Autodesk Inventor part; units mm, degrees
ref_plane "YZ Plane" through (0, 0, 0) normal (1, 0, 0) x (0, 1, 0)
ref_plane "XZ Plane" through (0, 0, 0) normal (0, 1, 0) x (-1, 0, 0)
ref_plane "XY Plane" through (0, 0, 0) normal (0, 0, 1) x (1, 0, 0)
sketch "Sketch1" plane through (0, 0, 0) normal (1, 0, 0) x (0, 1, 0)
  circle A0 centre (0, 0) radius 13.5
  dimension "d0" = 27
extrude "Extrusion1" add sketch "Sketch1" along normal blind 106
sketch "Sketch2" plane through (106, 0, 0) normal (1, 0, 0) x (0, 0, -1)
  circle A0 centre (0, 0) radius 1.5
  dimension "d3" = 3
extrude "Extrusion2" add sketch "Sketch2" along normal blind 12 and the other way blind 112.25
properties part number "ROLLER"
Source: CAD feature listing. Evaluate the final solid. Frame: model axes, mm. A direction names the side the tool comes from. Coordinates: 2 decimals unless noted, no trailing zeros. Loops run counter-clockwise (first coordinate to the right, second up) from the corner with the lowest first, then second, coordinate; pieces in that order, holes last. Notation, with made-up numbers: M 34,2 L 69,2 A20 cw 69,39 Z; hole C -30.75,-39 d8. An arc over 180 degrees is marked long. Put each result on its own line as item: value. Start each with the question number.
1) Cut plane A-A on y = 0. Return the cut outline in (x, z), then the cut area to 3 significant figures.
2) Cut plane C-C on x = 22. Return the cut outline in (y, z).
3) Cut plane D-D on y = 8.75. Return the cut outline in (x, z), then the cut area to 3 significant figures.
4) Pull-direction query (Z, two-part tool) for faces 1 (the face through (0, 3, 0)), 2 (the face through (111.92, -0.07, 1.5)); classes: pulls with the +Z half, pulls with the -Z half, needs draft (parallel to the pull), parting line crosses it, or undercut.
5) Reachability of faces 3 (the face through (52.26, -2.93, 13.18)), 4 (the face through (-3.08, 0.07, 1.5)) from +Z, -Z, +X, -X, +Y, -Y: full face, straight path, thin tool, end or side. Return the list, or none.
6) Ray query, L1, parallel to X at y = 7.75, z = -7.75; L2, parallel to Z at x = 105.5, y = -0.75; L3, parallel to Z at x = 89.5, y = -7.5. Return the intervals inside material, ascending. Write a range as from..to.
7) Contact query for flat-ended pins moving along their axis: pin 1 Ø8 at (y, z) = (4, 7) entering from -X; pin 2 Ø2 at (x, y) = (94.5, -8.5) entering from -Z (3 decimals); pin 3 Ø6 at (y, z) = (-8, 8.5) entering from +X. Output: stop coordinate, or through.
The answers:
1. outline: M -6.25,-1.5 L 0,-1.5 L 0,-13.5 L 106,-13.5 L 106,-1.5 L 118,-1.5 L 118,1.5 L 106,1.5 L 106,13.5 L 0,13.5 L 0,1.5 L -6.25,1.5 Z
1. area: 2,920 mm²
2. outline: C 0,0 d27
3. outline: M 0,-10.28 L 106,-10.28 L 106,10.28 L 0,10.28 Z
3. area: 2,180 mm²
4. face 1: needs draft
4. face 2: parting line crosses it
5. face 3: +X, -X
5. face 4: -X
6. L1: x = 0..106
6. L2: z = -13.48..13.48
6. L3: z = -11.22..11.22
7. pin 1: stops at x = 0
7. pin 2: stops at z = -11.225
7. pin 3: stops at x = 106
